from build123d import *

# Parameters (mm, degrees)
PAD_DEPTH       = 35
FILLET_R        = 25
SKETCH001_W     = 28
SKETCH001_H     = 35
PAD001_DEPTH    = 1
PAD002_DEPTH    = 28
SKETCH004_R     = 9.55
POCKET_DEPTH    = 35
SKETCH005_R     = 2.1
POCKET001_DEPTH = 69.001
FILLET001_R     = 6
FILLET002_R     = 2
FILLET003_R     = 3
FILLET004_R     = 6


with BuildPart() as part:
    # Sketch → Pad (new body)
    with BuildSketch(Plane.XY):
        with BuildLine():
            ThreePointArc((15, 64), (0, 76.46889), (-15, 64))
            ThreePointArc((-46.461169, -5.570082), (-26.519858, 27.310773), (-15, 64))
            ThreePointArc((-46.461169, -5.570082), (-50.972801, -47.763847), (-15, -70.272205))
            Line((-15, -70.272205), (15, -70.272205))
            ThreePointArc((15, -70.272205), (50.972801, -47.763847), (46.461169, -5.570082))
            ThreePointArc((15, 64), (26.519858, 27.310773), (46.461169, -5.570082))
        make_face()
    extrude(amount=PAD_DEPTH)

    # Fillet
    fillet_edges = [part.edges().sort_by_distance(p)[0] for p in [
        (0, 76.46889, 35),
    ]]
    fillet(fillet_edges, radius=FILLET_R)

    # Sketch001 → Pad001 (new body)
    with BuildSketch(Plane(origin=(0, 0, 0), x_dir=(1, 0, 0), z_dir=(0, 0, -1))):
        with Locations((0, 7.5)):
            Rectangle(SKETCH001_W, SKETCH001_H)
    extrude(amount=PAD001_DEPTH)

    # Sketch002 → Pad002 (new body)
    with BuildSketch(Plane.YZ.offset(14)):
        Polygon((-25, 0), (-19.152566, -19.126095), (10, -10.213261), (10, 0), align=None)
    extrude(amount=-PAD002_DEPTH)

    # Sketch004 → Pocket (cut)
    with BuildSketch(Plane(origin=(0, 3.710404, -12.136184), x_dir=(1, 0, 0), z_dir=(0, 0.292372, -0.956305))):
        with Locations((0, 8.66532)):
            Circle(SKETCH004_R)
    extrude(amount=-POCKET_DEPTH, mode=Mode.SUBTRACT)

    # Sketch005 → Pocket001 (cut, through all)
    with BuildSketch(Plane.YZ.offset(14)):
        with Locations((-6.769071, -7.497393)):
            Circle(SKETCH005_R)
    extrude(amount=-POCKET001_DEPTH, mode=Mode.SUBTRACT)

    # Fillet001
    fillet001_edges = [part.edges().sort_by_distance(p)[0] for p in [
        (14, 10, -5.606631),
        (-14, 10, -5.606631),
        (-14, -21.923418, -10.063048),
        (14, -21.923418, -10.063048),
    ]]
    fillet(fillet001_edges, radius=FILLET001_R)

    # Fillet002
    fillet002_edges = [part.edges().sort_by_distance(p)[0] for p in [
        (14, -4.707369, -14.709755),
    ]]
    fillet(fillet002_edges, radius=FILLET002_R)

    # Fillet003
    fillet003_edges = [part.edges().sort_by_distance(p)[0] for p in [
        (26.519858, 27.310773, 0),
    ]]
    fillet(fillet003_edges, radius=FILLET003_R)

    # Fillet004
    fillet004_edges = [part.edges().sort_by_distance(p)[0] for p in [
        (-14, -25, -0.5),
        (14, -25, -0.5),
    ]]
    fillet(fillet004_edges, radius=FILLET004_R)


solid = part.part
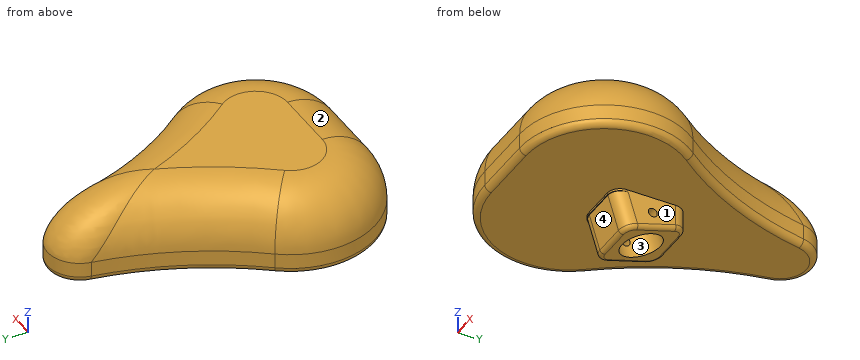
Geometry check sheet. Reference: the model listing, model coordinates, mm. Face numbers are marked on the shaded views. Round coordinates to 2 decimals unless told otherwise and drop trailing zeros. Answer in a Markdown table with one row per item. Add a question column.
Item 1: Draft check along Z on the marked faces 1, 2, 3 and 4. Enter one of: released by +Z, released by -Z, zero draft, split by the parting line, or undercut.
Item 2: Material ranges on L1, parallel to X at y = -13.5, z = 14; L2, parallel to Y at x = 44.5, z = 24; L3, parallel to X at y = 55.5, z = 9.5, recorded low to high. Write a range as [from, to].
Item 3: Depth check by flat-ended pin: pin 1 Ø1.5 at (x, z) = (1.5, 5) entering from +Y; pin 2 Ø4 at (y, z) = (-23, 28) entering from +X; pin 3 Ø6 at (y, z) = (2, 12.5) entering from -X; pin 4 Ø4 at (y, z) = (-6.77, -7.5) entering from -X. Enter the tip coordinate at first touch or a pass-through.
Filled in:
| question | item | result |
|---|---|---|
| 1 | face 1 | zero draft |
| 1 | face 2 | released by +Z |
| 1 | face 3 | undercut |
| 1 | face 4 | released by -Z |
| 2 | L1 | x = [-50.96, -9.55], [9.55, 50.96] |
| 2 | L2 | y = [-50.4, -10.14] |
| 2 | L3 | x = [-16.82, 16.82] |
| 3 | pin 1 | stops at y = 76.45 |
| 3 | pin 2 | stops at x = 48.48 |
| 3 | pin 3 | stops at x = -42.87 |
| 3 | pin 4 | passes through |
